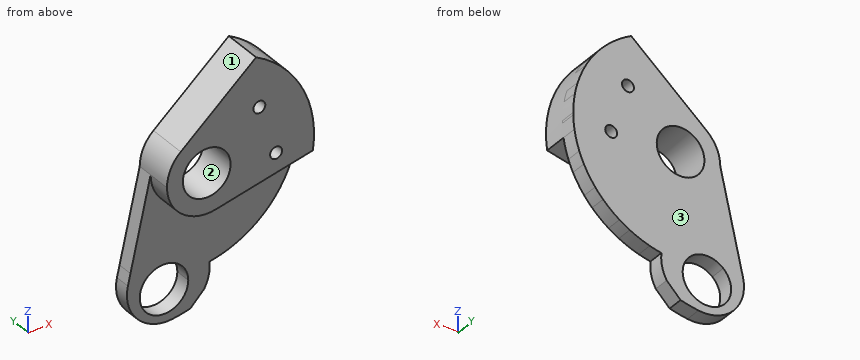
```python
from build123d import *

# Parameters (mm, degrees)
SKETCH_1_R      = 6
SKETCH_1_R_2    = 1.5
EXTRUDE_1_DEPTH = 4
EXTRUDE_START   = -10
SKETCH_2_R      = 6
SKETCH_2_R_2    = 1.5
EXTRUDE_3_DEPTH = 10


with BuildPart() as part:
    # 草图1 → 凸台-拉伸1 (new body)
    # profile 1 of 2: a face of its own
    with BuildSketch(Plane(origin=(0, 0, 0), x_dir=(1, 0, 0), z_dir=(0, 1, 0))):
        with BuildLine():
            ThreePointArc((-11.882996945, 32.788243467), (-20.67500257, 29.68936306), (-23.090953179, 20.685719055))
            Line((-23.090953179, 20.685719055), (-22.448063756, 17.847212503))
            ThreePointArc((-22.448063756, 17.847212503), (-20.341934216, 19.128766183), (-18.127687059, 20.212865348))
            ThreePointArc((-18.127687059, 20.212865348), (-16.454907522, 30.290305128), (-7.901384252, 24.70548431))
            ThreePointArc((-7.901384252, 24.70548431), (-8.01255227, 23.54622097), (-8.342004413, 22.429211075))
            ThreePointArc((-8.342004413, 22.429211075), (-5.436219765, 22.37688115), (-2.552893168, 22.012531633))
            ThreePointArc((-2.552893168, 22.012531633), (-2.714933584, 25.241816969), (-3.873838396, 28.260339871))
            Line((-3.873838396, 28.260339871), (-7.3745684, 31.841047256))
            ThreePointArc((-7.3745684, 31.841047256), (-9.61431765, 32.383495426), (-11.882996945, 32.788243467))
        make_face()
    # profile 2 of 2: a face of its own
    with BuildSketch(Plane(origin=(0, 0, 0), x_dir=(1, 0, 0), z_dir=(0, 1, 0))):
        with BuildLine():
            ThreePointArc((-18.127687059, 20.212865348), (-20.341934216, 19.128766183), (-22.448063756, 17.847212503))
            Line((-22.448063756, 17.847212503), (-17.3745684, -4.553451276))
            ThreePointArc((-17.3745684, -4.553451276), (-16.46911872, -8.71147418), (-13.916737505, -12.116520983))
            Line((-13.916737505, -12.116520983), (5.051344821, -28.524197627))
            ThreePointArc((5.051344821, -28.524197627), (7.070533196, -27.364392508), (8.982279547, -26.034920622))
            ThreePointArc((8.982279547, -26.034920622), (10.160528905, -25.084412347), (11.283653654, -24.069361447))
            ThreePointArc((11.283653654, -24.069361447), (13.156392672, -22.088548581), (14.819857518, -19.928998687))
            ThreePointArc((14.819857518, -19.928998687), (15.646716038, -18.660912524), (16.40120317, -17.348477117))
            ThreePointArc((16.40120317, -17.348477117), (17.570178978, -14.88590395), (18.484890443, -12.318011044))
            ThreePointArc((18.484890443, -12.318011044), (18.879419451, -10.8564761), (19.19141451, -9.375126508))
            ThreePointArc((19.19141451, -9.375126508), (19.516708425, -6.974036065), (19.6254316, -4.553451276))
            ThreePointArc((19.6254316, -4.553451276), (19.623728487, -4.250193605), (19.618619362, -3.946974192))
            ThreePointArc((19.618619362, -3.946974192), (19.542199611, -2.435055692), (19.381162346, -0.929796734))
            ThreePointArc((19.381162346, -0.929796734), (18.879419451, 1.749573548), (18.110066991, 4.364696458))
            ThreePointArc((18.110066991, 4.364696458), (17.570178978, 5.779001398), (16.951872839, 7.160824487))
            ThreePointArc((16.951872839, 7.160824487), (15.646716038, 9.554009971), (14.106900946, 11.80339667))
            ThreePointArc((14.106900946, 11.80339667), (13.156392672, 12.981646029), (12.141341771, 14.104770777))
            ThreePointArc((12.141341771, 14.104770777), (10.160528905, 15.977509795), (8.000979011, 17.640974641))
            ThreePointArc((8.000979011, 17.640974641), (6.732892848, 18.467833161), (5.420457441, 19.222320294))
            ThreePointArc((5.420457441, 19.222320294), (2.957884274, 20.391296102), (0.389991368, 21.306007566))
            ThreePointArc((0.389991368, 21.306007566), (-1.071543576, 21.700536575), (-2.552893168, 22.012531633))
            ThreePointArc((-2.552893168, 22.012531633), (-5.436219765, 22.37688115), (-8.342004413, 22.429211075))
            ThreePointArc((-8.342004413, 22.429211075), (-12.653931695, 18.756167408), (-18.127687059, 20.212865348))
        make_face()
        with Locations(Location((-7.3745684, -4.553451276, 0), (0, 0, 270))):
            Circle(SKETCH_1_R, mode=Mode.SUBTRACT)
        with Locations(Location((5.860803588, -16.002247211, 0), (0, 0, 270))):
            Circle(SKETCH_1_R_2, mode=Mode.SUBTRACT)
        with Locations(Location((10.079774126, -3.290151234, 0), (0, 0, 270))):
            Circle(SKETCH_1_R_2, mode=Mode.SUBTRACT)
    extrude(amount=EXTRUDE_1_DEPTH)

    # 草图2 → 凸台-拉伸3 (add)
    # profile 1 of 2: a face of its own
    with BuildSketch(Plane(origin=(0, 4, 0), x_dir=(1, 0, 0), z_dir=(0, 1, 0)).offset(EXTRUDE_START)):
        with BuildLine():
            ThreePointArc((2.6254316, -4.553451276), (0.461357134, 1.659299405), (-5.094222606, 5.183079064))
            ThreePointArc((-5.094222606, 5.183079064), (-13.587319081, 3.282474258), (-17.3745684, -4.553451276))
            ThreePointArc((-17.3745684, -4.553451276), (-16.46911872, -8.71147418), (-13.916737505, -12.116520983))
            ThreePointArc((-13.916737505, -12.116520983), (-3.216545495, -13.648001596), (2.6254316, -4.553451276))
        make_face()
        with Locations(Location((-7.3745684, -4.553451276, 0), (0, 0, 270))):
            Circle(SKETCH_2_R, mode=Mode.SUBTRACT)
    # profile 2 of 2: a face of its own
    with BuildSketch(Plane(origin=(0, 4, 0), x_dir=(1, 0, 0), z_dir=(0, 1, 0)).offset(EXTRUDE_START)):
        with BuildLine():
            Line((19.324871256, -0.535999093), (-5.094222606, 5.183079064))
            ThreePointArc((-5.094222606, 5.183079064), (0.461357134, 1.659299405), (2.6254316, -4.553451276))
            ThreePointArc((2.6254316, -4.553451276), (-3.216545495, -13.648001596), (-13.916737505, -12.116520983))
            Line((-13.916737505, -12.116520983), (5.051344821, -28.524197627))
            ThreePointArc((5.051344821, -28.524197627), (16.678147117, -16.819945325), (19.324871256, -0.535999093))
        make_face()
        with Locations(Location((5.860803588, -16.002247211, 0), (0, 0, 270))):
            Circle(SKETCH_2_R_2, mode=Mode.SUBTRACT)
        with Locations(Location((10.079774126, -3.290151234, 0), (0, 0, 270))):
            Circle(SKETCH_2_R_2, mode=Mode.SUBTRACT)
    extrude(amount=EXTRUDE_3_DEPTH)


solid = part.part
```
Could you check a few things on this model? Use its own coordinates, in mm. Face numbers are marked on the shaded views. Give positions to 0.01 mm unless a question says otherwise; leave off trailing zeros. Order: outer loops, then holes, each group sorted by start corner. A loop starts at its lowest first (then second) coordinate and runs counter-clockwise, first axis right, second up.
Q1. Suppose I cut it at C-C, the plane x = 15.5. Write out the boundary of the cut face in (y, z).
Q2. Suppose I cut it at B-B, the plane z = 7. Write out the boundary of the cut face in (x, y), and give its area (3 significant figures).
Q3. If I drill on line 1 along X through (y, z) = (-2, 3); line 2 along X through (y, z) = (2.25, -24); line 3 along X through (y, z) = (-1.5, 2), over which ranges is the centre line in solid material (lowest first)?
Q4. I'm going to push flat-ended pins straight in: P1, Ø11, axis at x = 0, z = -19.5, coming from the -Y side; P2, Ø1.5, axis at x = 12, y = -3.5, coming from the -Z side; P3, Ø2, axis at y = -4, z = 9, coming from the +X side. Where does each tip first touch, or does it pass through?
Q5. We'd pull the mould along Z, two halves only. Please class the marked faces 1, 2 and 3: +Z half, -Z half, draft (parallel to the pull), parting line (faces both ways), or undercut.
Q6. Suppose I cut it at A-A, the plane y = 1.75. Write out the boundary of the cut face in (x, z), and give its area (3 significant figures).
Q7. Suppose I cut it at D-D, the plane y = -4. Write out the boundary of the cut face in (x, z).
Solution:
1. outline: (-6, -0.36) - (0, -0.36) - (0, -9.79) - (4, -9.79) - (4, 18.9) - (-6, 18.9) - close
2. outline: (-17.07, -6) - (-12.85, -6) - (-12.85, 4) - (-17.07, 4) - close; (-1.9, -6) - (19.51, -6) - (19.51, 4) - (-1.9, 4) - close
2. area: 256 mm2
3. line 1: x = -17.25 to -13.17, -1.58 to 8.61, 11.55 to 19.58
3. line 2: x = -23.28 to -20.06, -7.94 to -2.53
3. line 3: x = -17.04 to -12.8, -1.95 to 9.31, 10.84 to 19.5
4. P1: stops at y = 0
4. P2: stops at z = -1.36
4. P3: stops at x = 19.4
5. face 1: +Z half
5. face 2: undercut
5. face 3: draft
6. outline: (-23.09, -20.69) arc R10 ccw to (-11.88, -32.79) arc R37.74 ccw to (-7.37, -31.84) - (-3.87, -28.26) arc R10.26 ccw to (-2.55, -22.01) arc R27 ccw to (19.62, 3.95) arc R27 ccw to (19.63, 4.55) arc R27 ccw to (5.05, 28.52) - (-13.92, 12.12) arc R10 ccw to (-17.37, 4.55) - close; hole circle Ø12.2 at (-14, -24.71); hole circle Ø12 at (-7.37, 4.55); hole circle Ø3 at (5.86, 16); hole circle Ø3 at (10.08, 3.29)
6. area: 1,420 mm2
7. outline: (-13.92, 12.12) arc R10 ccw to (-5.09, -5.18) - (19.32, 0.54) arc R27 ccw to (5.05, 28.52) - close; hole circle Ø12 at (-7.37, 4.55); hole circle Ø3 at (5.86, 16); hole circle Ø3 at (10.08, 3.29)
